Geometry: final body of the model. Coordinates: model frame, mm. A direction names the side the tool comes from. Give positions to 0.01 mm unless a question says otherwise; leave off trailing zeros. Loops run counter-clockwise (first coordinate to the right, second up) from the corner with the lowest first, then second, coordinate; pieces in that order, holes last. Notation, with made-up numbers: (-28, 31.25) - (-16, 31.25) arc R11 ccw to (-16, 35.25) - close; hole circle Ø11 at (-33, 52). An arc over 180 degrees is marked (long way). Use one line per item in the form item = value.
```python
from build123d import *

# Parameters (mm, degrees)
CYLINDER010_R     = 1.7
CYLINDER010_DEPTH = 10
CYLINDER009_R     = 1.7
CYLINDER009_DEPTH = 10
CYLINDER008_R     = 1.7
CYLINDER008_DEPTH = 10
CYLINDER007_R     = 1.7
CYLINDER007_DEPTH = 10
CYLINDER006_R     = 1.7
CYLINDER006_DEPTH = 10
CYLINDER005_R     = 1.7
CYLINDER005_DEPTH = 10
CYLINDER004_R     = 1.7
CYLINDER004_DEPTH = 10
CYLINDER003_R     = 1.7
CYLINDER003_DEPTH = 10
CYLINDER002_R     = 1.7
CYLINDER002_DEPTH = 10
CYLINDER001_R     = 1.7
CYLINDER001_DEPTH = 10
CYLINDER_R        = 1.7
CYLINDER_DEPTH    = 10
BOX007_W          = 41
BOX007_H          = 41
BOX007_DEPTH      = 3
BOX006_W          = 10
BOX006_H          = 25
BOX006_DEPTH      = 22
BOX005_W          = 10
BOX005_H          = 25
BOX005_DEPTH      = 22
BOX004_W          = 29
BOX004_H          = 23
BOX004_DEPTH      = 34
BOX004_ROLL_ANGLE = 45
BOX001_W          = 29
BOX001_H          = 25
BOX001_DEPTH      = 18
BOX003_W          = 10
BOX003_H          = 40
BOX003_DEPTH      = 3
BOX002_W          = 10
BOX002_H          = 40
BOX002_DEPTH      = 3
BOX_W             = 29
BOX_H             = 35
BOX_DEPTH         = 49


with BuildPart() as cylinder010:
    # Cylinder010 → Cylinder010 (new body)
    with BuildSketch(Plane(origin=(32, 2, 41), x_dir=(1, 0, 0), z_dir=(0, 0, 1))):
        Circle(CYLINDER010_R)
    extrude(amount=CYLINDER010_DEPTH)


with BuildPart() as cylinder009:
    # Cylinder009 → Cylinder009 (new body)
    with BuildSketch(Plane(origin=(32, 12, 41), x_dir=(1, 0, 0), z_dir=(0, 0, 1))):
        Circle(CYLINDER009_R)
    extrude(amount=CYLINDER009_DEPTH)


with BuildPart() as cylinder008:
    # Cylinder008 → Cylinder008 (new body)
    with BuildSketch(Plane(origin=(32, 22, 41), x_dir=(1, 0, 0), z_dir=(0, 0, 1))):
        Circle(CYLINDER008_R)
    extrude(amount=CYLINDER008_DEPTH)


with BuildPart() as cylinder007:
    # Cylinder007 → Cylinder007 (new body)
    with BuildSketch(Plane(origin=(32, 32, 41), x_dir=(1, 0, 0), z_dir=(0, 0, 1))):
        Circle(CYLINDER007_R)
    extrude(amount=CYLINDER007_DEPTH)


with BuildPart() as cylinder006:
    # Cylinder006 → Cylinder006 (new body)
    with BuildSketch(Plane(origin=(-3, 2, 41), x_dir=(1, 0, 0), z_dir=(0, 0, 1))):
        Circle(CYLINDER006_R)
    extrude(amount=CYLINDER006_DEPTH)


with BuildPart() as cylinder005:
    # Cylinder005 → Cylinder005 (new body)
    with BuildSketch(Plane(origin=(-3, 12, 41), x_dir=(1, 0, 0), z_dir=(0, 0, 1))):
        Circle(CYLINDER005_R)
    extrude(amount=CYLINDER005_DEPTH)


with BuildPart() as cylinder004:
    # Cylinder004 → Cylinder004 (new body)
    with BuildSketch(Plane(origin=(-3, 22, 41), x_dir=(1, 0, 0), z_dir=(0, 0, 1))):
        Circle(CYLINDER004_R)
    extrude(amount=CYLINDER004_DEPTH)


with BuildPart() as cylinder003:
    # Cylinder003 → Cylinder003 (new body)
    with BuildSketch(Plane(origin=(-3, 32, 41), x_dir=(1, 0, 0), z_dir=(0, 0, 1))):
        Circle(CYLINDER003_R)
    extrude(amount=CYLINDER003_DEPTH)


with BuildPart() as cylinder002:
    # Cylinder002 → Cylinder002 (new body)
    with BuildSketch(Plane(origin=(24, -3, 41), x_dir=(1, 0, 0), z_dir=(0, 0, 1))):
        Circle(CYLINDER002_R)
    extrude(amount=CYLINDER002_DEPTH)


with BuildPart() as cylinder001:
    # Cylinder001 → Cylinder001 (new body)
    with BuildSketch(Plane(origin=(5, -3, 41), x_dir=(1, 0, 0), z_dir=(0, 0, 1))):
        Circle(CYLINDER001_R)
    extrude(amount=CYLINDER001_DEPTH)


with BuildPart() as cylinder:
    # Cylinder → Cylinder (new body)
    with BuildSketch(Plane(origin=(14.5, -3, 41), x_dir=(1, 0, 0), z_dir=(0, 0, 1))):
        Circle(CYLINDER_R)
    extrude(amount=CYLINDER_DEPTH)


with BuildPart() as cut016:
    # Box007 → Box007 (new body)
    with BuildSketch(Plane(origin=(-6, -6, 46), x_dir=(1, 0, 0), z_dir=(0, 0, 1))):
        with Locations((20.5, 20.5)):
            Rectangle(BOX007_W, BOX007_H)
    extrude(amount=BOX007_DEPTH)

    # Cut006: cut Cylinder
    add(cylinder.part, mode=Mode.SUBTRACT)

    # Cut007: cut Cylinder001
    add(cylinder001.part, mode=Mode.SUBTRACT)

    # Cut008: cut Cylinder002
    add(cylinder002.part, mode=Mode.SUBTRACT)

    # Cut009: cut Cylinder003
    add(cylinder003.part, mode=Mode.SUBTRACT)

    # Cut010: cut Cylinder004
    add(cylinder004.part, mode=Mode.SUBTRACT)

    # Cut011: cut Cylinder005
    add(cylinder005.part, mode=Mode.SUBTRACT)

    # Cut012: cut Cylinder006
    add(cylinder006.part, mode=Mode.SUBTRACT)

    # Cut013: cut Cylinder007
    add(cylinder007.part, mode=Mode.SUBTRACT)

    # Cut014: cut Cylinder008
    add(cylinder008.part, mode=Mode.SUBTRACT)

    # Cut015: cut Cylinder009
    add(cylinder009.part, mode=Mode.SUBTRACT)

    # Cut016: cut Cylinder010
    add(cylinder010.part, mode=Mode.SUBTRACT)


with BuildPart() as cube006:
    # Box006 → Box006 (new body)
    with BuildSketch(Plane(origin=(16, 0, 24), x_dir=(1, 0, 0), z_dir=(0, 0, 1))):
        with Locations((5, 12.5)):
            Rectangle(BOX006_W, BOX006_H)
    extrude(amount=BOX006_DEPTH)


with BuildPart() as cube005:
    # Box005 → Box005 (new body)
    with BuildSketch(Plane(origin=(3, 0, 24), x_dir=(1, 0, 0), z_dir=(0, 0, 1))):
        with Locations((5, 12.5)):
            Rectangle(BOX005_W, BOX005_H)
    extrude(amount=BOX005_DEPTH)


with BuildPart() as cube004:
    # Box004 → Box004 (new body)
    with BuildSketch(Plane.XY):
        with Locations((14.5, 11.5)):
            Rectangle(BOX004_W, BOX004_H)
    extrude(amount=BOX004_DEPTH)


with BuildPart() as cube004_1:
    # Box004 roll: moved
    add(cube004.part.rotate(Axis((0, 0, 0), (1, 0, 0)), BOX004_ROLL_ANGLE))


with BuildPart() as cube004_2:
    # Box004 placement: moved
    add(cube004_1.part.moved(Location((0, 7, 7))))


with BuildPart() as cube001:
    # Box001 → Box001 (new body)
    with BuildSketch(Plane.XY.offset(6)):
        with Locations((14.5, 12.5)):
            Rectangle(BOX001_W, BOX001_H)
    extrude(amount=BOX001_DEPTH)


with BuildPart() as cube003:
    # Box003 → Box003 (new body)
    with BuildSketch(Plane(origin=(16, 0, 0), x_dir=(1, 0, 0), z_dir=(0, 0, 1))):
        with Locations((5, 20)):
            Rectangle(BOX003_W, BOX003_H)
    extrude(amount=BOX003_DEPTH)


with BuildPart() as cube002:
    # Box002 → Box002 (new body)
    with BuildSketch(Plane(origin=(3, 0, 0), x_dir=(1, 0, 0), z_dir=(0, 0, 1))):
        with Locations((5, 20)):
            Rectangle(BOX002_W, BOX002_H)
    extrude(amount=BOX002_DEPTH)


with BuildPart() as fusion:
    # Box → Box (new body)
    with BuildSketch(Plane.XY):
        with Locations((14.5, 17.5)):
            Rectangle(BOX_W, BOX_H)
    extrude(amount=BOX_DEPTH)

    # Cut: cut Cube002
    add(cube002.part, mode=Mode.SUBTRACT)

    # Cut001: cut Cube003
    add(cube003.part, mode=Mode.SUBTRACT)

    # Cut002: cut Cube001
    add(cube001.part, mode=Mode.SUBTRACT)

    # Cut003: cut Cube004
    add(cube004_2.part, mode=Mode.SUBTRACT)

    # Cut004: cut Cube005
    add(cube005.part, mode=Mode.SUBTRACT)

    # Cut005: cut Cube006
    add(cube006.part, mode=Mode.SUBTRACT)

    # Fusion: union Cut016
    add(cut016.part)


solid = fusion.part
```
(1) Material intervals for L1, parallel to X at y = -3, z = 47.3; L2, parallel to Y at x = 32, z = 46.9; L3, parallel to X at y = 32, z = 47.05, sorted ascending. Write a range as from..to.
Solution:
L1 = -6..3.3, 6.7..12.8, 16.2..22.3, 25.7..35
L2 = -6..0.3, 3.7..10.3, 13.7..20.3, 23.7..30.3, 33.7..35
L3 = -6..-4.7, -1.3..30.3, 33.7..35
(2) Pull-direction query (Z, two-part tool) for faces 1 (the face through (27, 18, 0)), 2 (the face through (16.07, -3.65, 47.48)), 3 (the face through (27, 24, 24)); classes: released by +Z, released by -Z, zero draft, split by the parting line, or undercut.
Solution:
face_1 = released by -Z
face_2 = zero draft
face_3 = undercut
(3) Cut plane B-B (y = 32). Return the cut outline in (x, z).
Solution:
outline = (-6, 46) - (-4.7, 46) - (-4.7, 49) - (-6, 49) - close; (-1.3, 46) - (0, 46) - (0, 0) - (3, 0) - (3, 3) - (13, 3) - (13, 0) - (16, 0) - (16, 3) - (26, 3) - (26, 0) - (29, 0) - (29, 46) - (30.3, 46) - (30.3, 49) - (-1.3, 49) - close; (33.7, 46) - (35, 46) - (35, 49) - (33.7, 49) - close
(4) Access query for faces 4 (the face through (0, 21, 28)), 5 (the face through (16, 15, 37)), 6 (the face through (16, 17, 1)). Directions: +Z, -Z, +X, -X, +Y, -Y. A direction counts if a zero-diameter tool reaches every point of the face in a straight line with its end or side. Return the directions, or none.
Solution:
face_4 = -Z, -X, +Y, -Y
face_5 = -Y
face_6 = -Z, +Y, -Y
(5) Cut plane C-C (x = 24). Return the cut outline in (y, z), plus the area to 3 significant figures.
Solution:
outline = (-6, 46) - (-4.7, 46) - (-4.7, 49) - (-6, 49) - close; (-1.3, 46) - (25, 46) - (25, 6) - (0, 6) - (0, 3) - (35, 3) - (35, 49) - (-1.3, 49) - close
area = 618 mm2
(6) Pin query (flat end, axial travel): P1, Ø4, axis at x = 19.5, z = 7, coming from the -Y side; P2, Ø8, axis at y = 21.5, z = 28.5, coming from the -X side; P3, Ø2, axis at y = 17.5, z = 30.5, coming from the +X side. Return the tip coordinate at first contact, or that it passes through.
Solution:
P1 = 0
P2 = 0
P3 = 29
(7) Cut plane D-D (x = -3). Return the cut outline in (y, z).
Solution:
outline = (-6, 46) - (0.3, 46) - (0.3, 49) - (-6, 49) - close; (3.7, 46) - (10.3, 46) - (10.3, 49) - (3.7, 49) - close; (13.7, 46) - (20.3, 46) - (20.3, 49) - (13.7, 49) - close; (23.7, 46) - (30.3, 46) - (30.3, 49) - (23.7, 49) - close; (33.7, 46) - (35, 46) - (35, 49) - (33.7, 49) - close
(8) Cut plane A-A (y = -3). Return the cut outline in (x, z), plus the area to 3 significant figures.
Solution:
outline = (-6, 46) - (3.3, 46) - (3.3, 49) - (-6, 49) - close; (6.7, 46) - (12.8, 46) - (12.8, 49) - (6.7, 49) - close; (16.2, 46) - (22.3, 46) - (22.3, 49) - (16.2, 49) - close; (25.7, 46) - (35, 46) - (35, 49) - (25.7, 49) - close
area = 92.4 mm2
